Source: CAD feature listing. Evaluate the final solid. Frame: model axes, mm. A direction names the side the tool comes from. Round coordinates to 2 decimals unless told otherwise and drop trailing zeros. Write each loop counter-clockwise with the first axis right and the second up, starting at its lowest first coordinate (ties: lowest second). Pieces come first, ordered by that corner, then holes. Notation, with made-up numbers: M 1.5,53 L 35.5,53 A18 ccw 35.5,63 Z; hole C -2.5,66 d3. An arc over 180 degrees is marked long. Answer in a Markdown table with one row per item. Add a question column.
Item 1: Cut plane A-A on z = 19. Return loops of the section in (x, y), and give its area (3 significant figures).
Item 2: Cut plane C-C on z = 25. Return loops of the section in (x, y), and give its area (3 significant figures).
Item 3: Material intervals for probe 1 along Z at (x, y) = (-50, 13); probe 2 along X at (y, z) = (26, 37); probe 3 along Z at (x, y) = (-49.7, 62.5), sorted ascending.
Item 4: Contact query for a flat-ended pin moving along its axis: pin 1 (3 mm diameter, centred on x = -46, z = 9, fed in from +Y). Output: stop coordinate, or through.
Item 5: Mould query, pull axis Z, two halves, no side actions, for faces 1 (the face through (-25.24, 2.54, 25.48)), 2 (the face through (-0.99, 35, 25)), 3 (the face through (-51, 13, 47)), 4 (the face through (-27, 4, 0)). Classes: released by +Z, released by -Z, zero draft, split by the parting line, or undercut.
Item 6: Cut plane B-B on y = 13. Return loops of the section in (x, z), and give its area (3 significant figures).
Item 7: Cut plane D-D on x = -34.5. Return loops of the section in (y, z), and give its area (3 significant figures).
Item 8: Set-up query: faces 5 (the face through (-48.714, 37, 25)), 6 (the face through (-27, 0, 25)), 7 (the face through (-51, 40, 18)). Return all of +Z, -Z, +X, -X, +Y, -Y with unobstructed straight access to the full face (end or side cutting, diameter ignored); none if empty.
from build123d import *

# Parameters (mm, degrees)
EXTRUDE_1_DEPTH          = 50
SKETCH_2_R               = 1
CUT_EXTRUDE_1_DEPTH      = 97.622978633
SKETCH_3_R               = 1.6
CUT_EXTRUDE_2_DEPTH      = 99.031557982
CUT_EXTRUDE_3_DEPTH      = 97.622978633
CUT_EXTRUDE_3_DEPTH_BACK = 97.622978633
SKETCH_4_R               = 3
EXTRUDE_2_DEPTH          = 50
SKETCH_6_R               = 3
CUT_EXTRUDE_4_DEPTH      = 100


with BuildPart() as part:
    # ｽｹｯﾁ1 → ﾎﾞｽ - 押し出し1 (new body)
    with BuildSketch(Plane.XY):
        Polygon((-53.713930785, 70), (-53.713930785, 0), (-4.713930785, 0), (-4.713930785, 5), (-48.713930785, 5), (-48.713930785, 70), align=None)
    extrude(amount=EXTRUDE_1_DEPTH)

    # ｽｹｯﾁ2 → ｶｯﾄ - 押し出し1 (cut, through all)
    with BuildSketch(Plane(origin=(-48.713930785, 0, 0), x_dir=(0, 0, -1), z_dir=(1, 0, 0))):
        with Locations(Location((-46, 40, 0), (0, 0, 90))):
            Circle(SKETCH_2_R)
        with Locations(Location((-19, 40, 0), (0, 0, 90))):
            Circle(SKETCH_2_R)
        with Locations(Location((-19, 13, 0), (0, 0, 90))):
            Circle(SKETCH_2_R)
        with Locations(Location((-46, 13, 0), (0, 0, 90))):
            Circle(SKETCH_2_R)
    extrude(amount=-CUT_EXTRUDE_1_DEPTH, mode=Mode.SUBTRACT)

    # ｽｹｯﾁ3 → ｶｯﾄ - 押し出し2 (cut, through all)
    with BuildSketch(Plane(origin=(0, 5, 0), x_dir=(1, 0, 0), z_dir=(0, 1, 0))):
        with Locations(Location((-38.713930785, -25, 0), (0, 0, 180))):
            Circle(SKETCH_3_R)
        with Locations(Location((-23.713930785, -25, 0), (0, 0, 180))):
            Circle(SKETCH_3_R)
    extrude(amount=-CUT_EXTRUDE_2_DEPTH, mode=Mode.SUBTRACT)

    # ｽｹｯﾁ4 → ｶｯﾄ - 押し出し3 (cut, two sides: drawn at the far end of the back side and taken through both)
    with BuildSketch(Plane(origin=(-48.713930785, 0, 0), x_dir=(0, 0, -1), z_dir=(1, 0, 0)).offset(-CUT_EXTRUDE_3_DEPTH_BACK)):
        with Locations((-32.5, 62.5)):
            Circle(SKETCH_4_R)
        with Locations((-12.5, 62.5)):
            Circle(SKETCH_4_R)
    extrude(amount=CUT_EXTRUDE_3_DEPTH + CUT_EXTRUDE_3_DEPTH_BACK, mode=Mode.SUBTRACT)

    # ｽｹｯﾁ5 → ﾎﾞｽ - 押し出し2 (add)
    with BuildSketch(Plane.XY.offset(50)):
        Polygon((-4.713930785, 5), (-4.713930785, 70), (-0.989780717, 70), (-0.989780717, 0), (-4.713930785, 0), align=None)
    extrude(amount=-EXTRUDE_2_DEPTH)

    # ｽｹｯﾁ6 → ｶｯﾄ - 押し出し4 (cut, through all)
    with BuildSketch(Plane.ZY.offset(4.713930785)):
        with Locations(Location((12.5, 62.5, 0), (0, 0, 180))):
            Circle(SKETCH_6_R)
        with Locations(Location((32.5, 62.5, 0), (0, 0, 180))):
            Circle(SKETCH_6_R)
    extrude(amount=-CUT_EXTRUDE_4_DEPTH, mode=Mode.SUBTRACT)


solid = part.part
Results below:
| question | item | result |
|---|---|---|
| 1 | outline | M -53.71,0 L -0.99,0 L -0.99,70 L -4.71,70 L -4.71,5 L -48.71,5 L -48.71,12 L -53.71,12 Z; M -53.71,14 L -48.71,14 L -48.71,39 L -53.71,39 Z; M -53.71,41 L -48.71,41 L -48.71,70 L -53.71,70 Z |
| 1 | area | 811 mm2 |
| 2 | outline | M -53.71,0 L -40.31,0 L -40.31,5 L -48.71,5 L -48.71,70 L -53.71,70 Z; M -37.11,0 L -25.31,0 L -25.31,5 L -37.11,5 Z; M -22.11,0 L -0.99,0 L -0.99,70 L -4.71,70 L -4.71,5 L -22.11,5 Z |
| 2 | area | 799 mm2 |
| 3 | probe 1 | 0 to 18, 20 to 45, 47 to 50 |
| 3 | probe 2 | -53.71 to -48.71, -4.71 to -0.99 |
| 3 | probe 3 | 0 to 9.5, 15.5 to 29.5, 35.5 to 50 |
| 4 | pin 1 | y = 5 |
| 5 | face 1 | undercut |
| 5 | face 2 | zero draft |
| 5 | face 3 | undercut |
| 5 | face 4 | released by -Z |
| 6 | outline | M -53.71,0 L -48.71,0 L -48.71,18 L -53.71,18 Z; M -53.71,20 L -48.71,20 L -48.71,45 L -53.71,45 Z; M -53.71,47 L -48.71,47 L -48.71,50 L -53.71,50 Z; M -4.71,0 L -0.99,0 L -0.99,50 L -4.71,50 Z |
| 6 | area | 416 mm2 |
| 7 | outline | M 0,0 L 5,0 L 5,50 L 0,50 Z |
| 7 | area | 250 mm2 |
| 8 | face 5 | +Z, -Z, +Y |
| 8 | face 6 | +Z, -Z, +X, -X, -Y |
| 8 | face 7 | -X |
